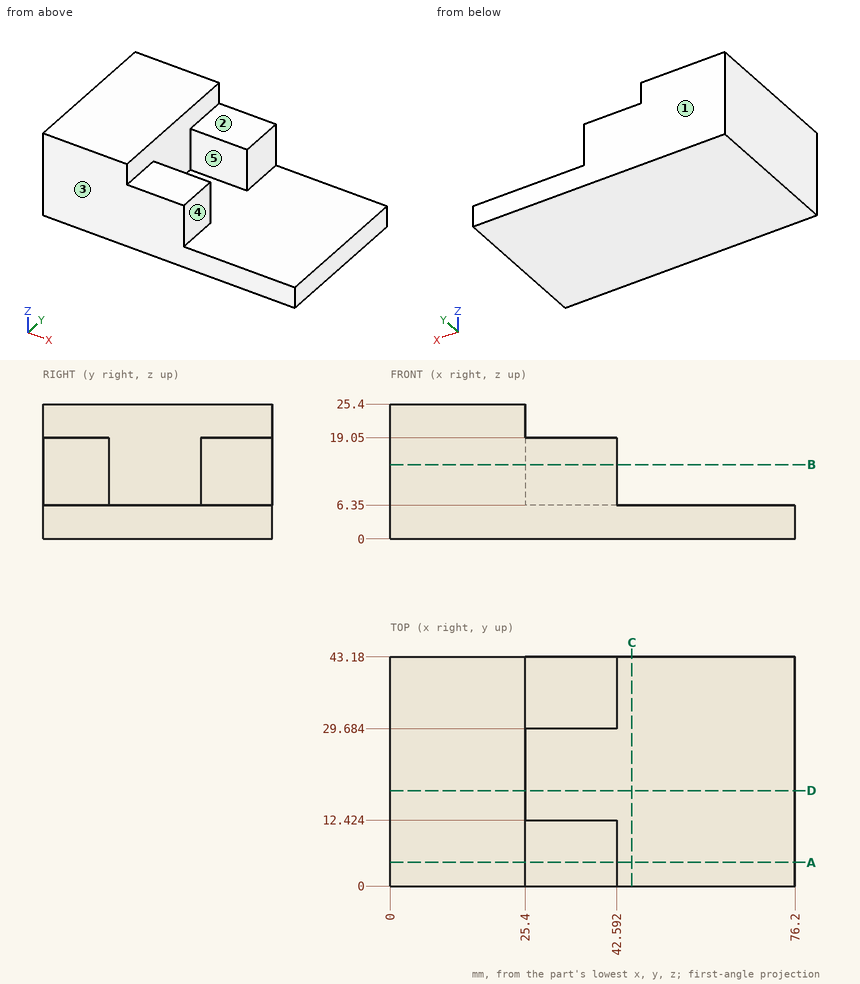
Study the drawing (mm; zero at the part's minimum x, y, z) and answer. A direction names the side the tool comes from. Give positions to 0.01 mm unless a question says otherwise; leave off trailing zeros. Loops run counter-clockwise (first coordinate to the right, second up) from the corner with the lowest first, then second, coordinate; pieces in that order, holes last. Notation, with made-up numbers: (11.25, 89.25) - (21.25, 89.25) arc R18 cw to (21.25, 116.25) - close; hole circle Ø1 at (-17, -6.5). An arc over 180 degrees is marked (long way). Answer as CSV lines item,"result". Start each with the question number.
1) Find section A-A (y = 4.5). Write down the section's boundary in (x, z).
2) Which of the six approach directions +Z, -Z, +X, -X, +Y, -Y give full straight-line access (tool end or side, diameter ignored) to the marked faces 1 and 2?
3) Find section C-C (x = 45.5). Write down the section's boundary in (y, z), then the cut area to 3 significant figures.
4) Each of these flat-tipped pins is pushed along its axis until it touches: pin 1 Ø5 at (x, y) = (54, 18.5) entering from +Z; pin 2 Ø2 at (y, z) = (29.5, 22) entering from +X; pin 3 Ø10 at (y, z) = (5, 10.5) entering from +X; pin 4 Ø8 at (x, y) = (41.5, 34) entering from +Z. Where does it stop, or does it pass through?
5) Find section D-D (y = 18). Write down the section's boundary in (x, z).
6) Straight lines are drawn through the part: L1, parallel to X at y = 2, z = 23.75; L2, parallel to Z at x = 34, y = 14; L3, parallel to Y at x = 40, z = 11.5 (1 decimal). For each, find the intervals that lie inside material, in ascending order. Write a range as from..to.
7) Find section B-B (z = 14). Write down the section's boundary in (x, y) (1 decimal), then the cut area to 3 significant figures.
8) Determine the mould class of the marked faces 3, 4 and 5 for opening direction Y: released by +Y, released by -Y, zero draft, split by the parting line, or undercut.
Findings below:
1,outline,"(0, 0) - (76.2, 0) - (76.2, 6.35) - (42.59, 6.35) - (42.59, 19.05) - (25.4, 19.05) - (25.4, 25.4) - (0, 25.4) - close"
2,face 1,"+Z, -Z, +X, -X, +Y"
2,face 2,"+Z, +X, +Y, -Y"
3,outline,"(0, 0) - (43.18, 0) - (43.18, 6.35) - (0, 6.35) - close"
3,area,"274 mm^2"
4,pin 1,"z = 6.35"
4,pin 2,"x = 25.4"
4,pin 3,"x = 76.2"
4,pin 4,"z = 19.05"
5,outline,"(0, 0) - (76.2, 0) - (76.2, 6.35) - (25.4, 6.35) - (25.4, 25.4) - (0, 25.4) - close"
6,L1,"0..25.4"
6,L2,"0..6.35"
6,L3,"0..12.4, 29.7..43.2"
7,outline,"(0, 0) - (42.6, 0) - (42.6, 12.4) - (25.4, 12.4) - (25.4, 29.7) - (42.6, 29.7) - (42.6, 43.2) - (0, 43.2) - close"
7,area,"1,540 mm^2"
8,face 3,"released by -Y"
8,face 4,"zero draft"
8,face 5,"undercut"
